Study the drawing (mm; zero at the part's minimum x, y, z) and answer. A direction names the side the tool comes from. Round coordinates to 2 decimals unless told otherwise and drop trailing zeros. Write each loop counter-clockwise with the first axis right and the second up, starting at its lowest first coordinate (ties: lowest second). Pieces come first, ordered by that corner, then holes. Notation, with made-up numbers: (77, 66.25) - (97, 66.25) arc R8 ccw to (97, 71.25) - close; hole circle Ø4 at (50, 11). An arc over 180 degrees is marked (long way). Use one line per item in the form item = value. Start each with the question number.
1) The part is cut by section D-D, the plane z = 0.65. Give the vertices of the cut face in (x, y).
2) The part is cut by section A-A, the plane z = 1.65. Give the vertices of the cut face in (x, y), plus the area to 3 significant figures.
3) The part is cut by section C-C, the plane y = 1.55. Give the vertices of the cut face in (x, z).
4) For the marked faces 5 and 6, determine the directions among +Z, -Z, +X, -X, +Y, -Y from which every point of the face is accessible in a straight line to the end or side of a thin tool.
5) For a pull along X with two mould halves and no side action, classify the marked faces 1, 2, 3 and 4 as released by +X, released by -X, zero draft, split by the parting line, or undercut.
6) The part is cut by section B-B, the plane x = 1.5. Give the vertices of the cut face in (y, z), plus the area to 3 significant figures.
7) Each of these flat-tipped pins is pushed along its axis until it touches: pin 1 (1.5 mm diameter, centred on x = 5, y = 3.5, fed in from +Z); pin 2 (3 mm diameter, centred on x = 1, z = 4.5, fed in from +Y); pin 3 (2 mm diameter, centred on y = 3.5, z = 3, fed in from -X); pin 4 (1.5 mm diameter, centred on x = 1, y = 5.5, fed in from -Z). Where does it stop, or does it pass through?
8) Consider line 1 along Z through (x, y) = (0.75, 1.9); line 2 along X through (y, z) = (4.7, 2.1); line 3 along Z through (x, y) = (3.75, 3.65). Determine where each line is inside the solid, lowest interval first. Write a range as from..to.
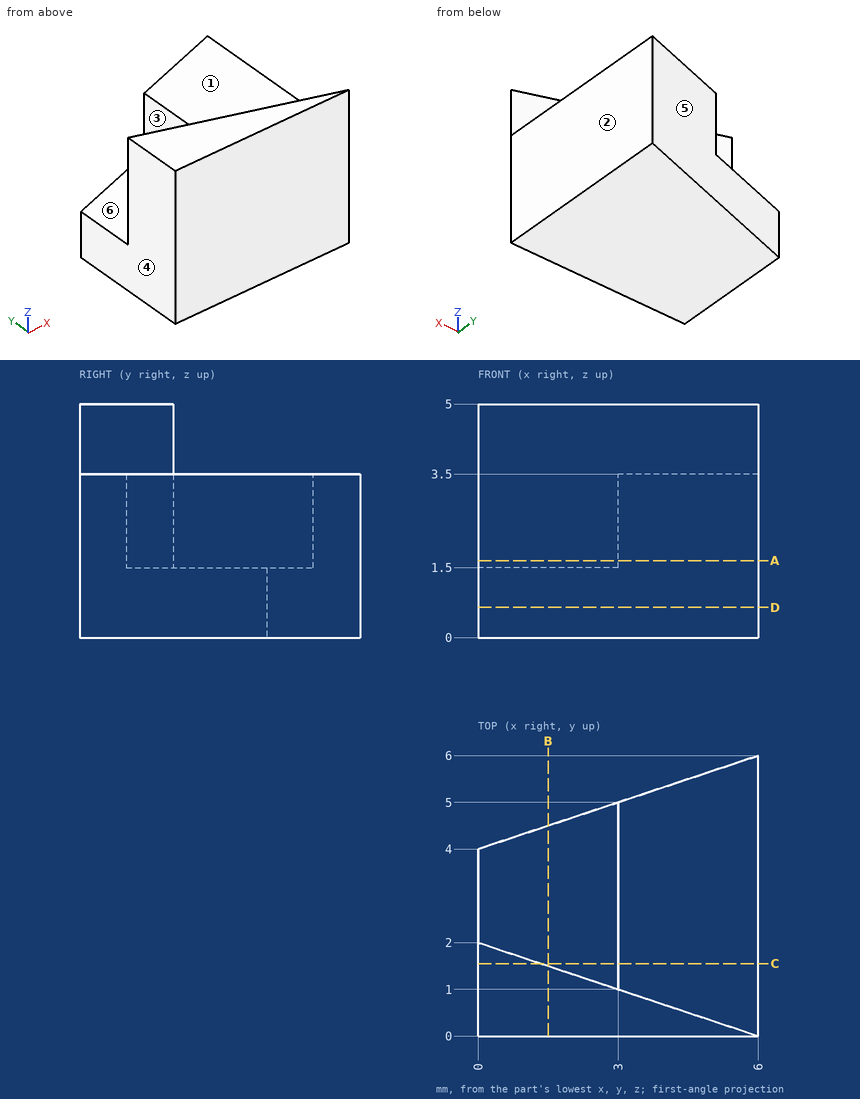
Geometry results:
q1.outline = (0, 0) - (6, 0) - (6, 6) - (0, 4) - close
q2.outline = (0, 0) - (6, 0) - (6, 6) - (3, 5) - (3, 1) - (0, 2) - close
q2.area = 21.0 mm2
q3.outline = (0, 0) - (6, 0) - (6, 3.5) - (3, 3.5) - (3, 1.5) - (1.35, 1.5) - (1.35, 5) - (0, 5) - close
q4.face_5 = +Z, -Z, -X, +Y
q4.face_6 = +Z, +Y
q5.face_1 = zero draft
q5.face_2 = released by +X
q5.face_3 = undercut
q5.face_4 = released by -X
q6.outline = (0, 0) - (4.5, 0) - (4.5, 1.5) - (1.5, 1.5) - (1.5, 5) - (0, 5) - close
q6.area = 12.0 mm2
q7.pin_1 = 3.5
q7.pin_2 = 2
q7.pin_3 = 3
q7.pin_4 = through
q8.line_1 = 0..1.5
q8.line_2 = 3..6
q8.line_3 = 0..3.5
